Build history of the part. All positions in model axes, mm. Face numbers are marked on the shaded views. A direction names the side the tool comes from. Round coordinates to 2 decimals unless told otherwise and drop trailing zeros. Write each loop counter-clockwise with the first axis right and the second up, starting at its lowest first coordinate (ties: lowest second). Pieces come first, ordered by that corner, then holes. Notation, with made-up numbers: (-6, 56) - (43, 56) arc R15 cw to (43, 66) - close; hole circle Ø10 at (-17, -4). An arc over 180 degrees is marked (long way). Write each question's results on one line, items separated by ' | '.
Autodesk Inventor part; units mm, degrees
ref_plane "YZ Plane" through (0, 0, 0) normal (1, 0, 0) x (0, 1, 0)
ref_plane "XZ Plane" through (0, 0, 0) normal (0, 1, 0) x (-1, 0, 0)
ref_plane "XY Plane" through (0, 0, 0) normal (0, 0, 1) x (1, 0, 0)
sketch "Sketch_1" plane through (0, 0, 0) normal (0, 0, 1) x (1, 0, 0)
  line L0 (0, 0) -> (0, 44)
  arc A0 (20.2731, 41) -> (0, 44) centre (0, -26) ccw
  line L1 (20.2731, 41) -> (22.5, 41)
  line L2 (22.5, 41) -> (23.5, 40)
  line L3 (23.5, 40) -> (23.5, 15.5)
  arc A1 (23, 15) -> (23.5, 15.5) centre (23, 15.5) ccw
  line L4 (23, 15) -> (19.5, 15)
  line L5 (19.5, 15) -> (19.5, 0.8)
  arc A2 (19, 0.3) -> (19.5, 0.8) centre (19, 0.8) ccw
  line L6 (19, 0.3) -> (4.5, 0.3)
  line L7 (4.5, 0.3) -> (4.5, 0)
  line L8 (4.5, 0) -> (0, 0)
  line L9 (0, 0) -> (0, 44)
revolve "Revolution1" add sketch "Sketch_1" angle 360 about axis through (0, 0, 0) along (0, -1, 0)
sketch "Sketch_2" plane through (0, 0, 0) normal (0, 0, 1) x (1, 0, 0)
  line L0 (0, -30) -> (0, 0)
  line L1 (0, 0) -> (3, 0)
  line L2 (3, 0) -> (3, -29.3865)
  line L3 (3, -29.3865) -> (2.3865, -30)
  line L4 (2.3865, -30) -> (0, -30)
  line L5 (0, -30) -> (0, 0)
revolve "Revolution2" add sketch "Sketch_2" angle 360 about axis through (0, -30, 0) along (0, -1, 0)
thread "Thread1"
properties part number "Torque limiting knob screw GN 5910-47-M6-30-1-SW"
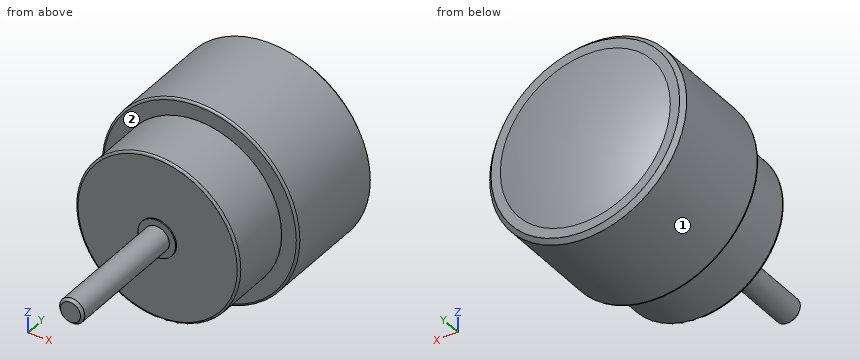
(1) Slice it at B-B, the plane y = 35. Write the cut outline in (x, z), and give its area (3 significant figures).
Worked answers:
outline: circle Ø47 at (0, 0) | area: 1,730 mm2
(2) Slice it at A-A, the plane y = 5. Write the cut outline in (x, z), and give its area (3 significant figures).
Worked answers:
outline: circle Ø39 at (0, 0) | area: 1,190 mm2
(3) Flat gauge pins, fed straight in: pin 1 Ø4 at (x, y) = (-17.5, 24) entering from -Z; pin 2 Ø4 at (x, y) = (18, 23.5) entering from -Z; pin 3 Ø1.5 at (y, z) = (20, 3.5) entering from -X. Where does each tip first touch, or does it go through?
Worked answers:
pin 1: stops at z = -17.66 | pin 2: stops at z = -17.21 | pin 3: stops at x = -23.34
(4) Tool access for the marked faces 1 and 2: list every direction of +Z, -Z, +X, -X, +Y, -Y with a clear straight run to the whole face (end or side of a thin tool).
Worked answers:
face 1: +Y, -Y | face 2: -Y
(5) Drill centre lines: probe 1 along Y at (x, z) = (-9, -18.5); probe 2 along X at (y, z) = (11, -3); probe 3 along X at (y, z) = (16, 20). Where is each one in solid material? Low to high. Write a range as [from, to].
Worked answers:
probe 1: y = [15, 41] | probe 2: x = [-19.27, 19.27] | probe 3: x = [-12.34, 12.34]
